Model file for the job. Use its own axes, mm. A direction names the side the tool comes from. Round coordinates to 2 decimals unless told otherwise and drop trailing zeros. Loops run counter-clockwise (first coordinate to the right, second up) from the corner with the lowest first, then second, coordinate; pieces in that order, holes last. Notation, with made-up numbers: M 2,-18.75 L 10,-18.75 A34 cw 10,16.25 Z; hole C -37.5,-31 d1. An arc over 180 degrees is marked long. Use a Markdown table: item, result. Add a question column.
Q1. Cut at D-D (z = -0.5). Give the cut face in (x, y).
Q2. Pin check, flat tip, straight feed: pin 1 (3 mm diameter, centred on x = 5, y = -3.5, fed in from -Z). Stop position of the tip, or through.
Q3. Cut at A-A (z = 0.3). Give the cut face in (x, y), plus the area to 3 significant figures.
Q4. Tool access for faces 1 (the face through (0, 0, -1.9)), 2 (the face through (-2, 2, 0.1)): list every direction of +Z, -Z, +X, -X, +Y, -Y with a clear straight run to the whole face (end or side of a thin tool).
Q5. Probe line 1 (Z direction, x = 4.5, y = 4); line 2 (X direction, y = -0.5, z = 0.15); line 3 (Y direction, x = -1, z = -0.4). List the from-to ranges inside material, lowest first. Write a range as from..to.
Q6. Cut at B-B (y = 5). Give the cut face in (x, z).
from build123d import *

# Parameters (mm, degrees)
F0_R            = 2.25
F1_DEPTH        = 2
F1_TAPER        = 3
F2_R            = 7
F3_DEPTH        = 0.5
F5_R            = 0.15
F6_DEPTH        = 0.1
F6_COPIES_COUNT = 4


# Not quite as in the source:
# - a pattern or mirror of a feature is missing from the dataset's text; its kind, count and spacing are read off the source's solid


with BuildPart() as f1:
    # F0 (on Top) → F1 (new body)
    with BuildSketch(Plane.XY):
        Circle(F0_R)
    extrude(amount=-F1_DEPTH, taper=F1_TAPER)

    # F2 (on Top) → F3 (join)
    with BuildSketch(Plane.XY):
        Circle(F2_R)
    extrude(amount=F3_DEPTH)


with BuildPart() as f1_1:
    # F4: moved
    add(f1.part.moved(Location((0, 0, 0.1))))

    # F5 (on Top) → F6 (join)
    with BuildSketch(Plane.XY):
        with Locations((-4, 0)):
            Circle(F5_R)
    f6 = extrude(amount=F6_DEPTH)

    # F6_copies: F6 ×4 about axis
    f6_copies_axis = Axis((0, 0, 0), (0, 0, 1))
    for i in range(1, F6_COPIES_COUNT):
        add(f6.rotate(f6_copies_axis, i * 360 / F6_COPIES_COUNT))


solid = f1_1.part
Checked values:
| question | item | result |
|---|---|---|
| 1 | outline | C 0,0 d4.44 |
| 2 | pin 1 | stops at z = 0.1 |
| 3 | outline | C 0,0 d14 |
| 3 | area | 154 mm^2 |
| 4 | face 1 | -Z, +X, -X, +Y, -Y |
| 4 | face 2 | -Z |
| 5 | line 1 | z = 0.1..0.6 |
| 5 | line 2 | x = -6.98..6.98 |
| 5 | line 3 | y = -1.99..1.99 |
| 6 | outline | M -4.9,0.1 L 4.9,0.1 L 4.9,0.6 L -4.9,0.6 Z |
